from build123d import *

# Parameters (mm, degrees)
SKETCH_1_W             = 60
SKETCH_1_H             = 80
EXTRUDE_1_DEPTH        = 23
SKETCH_3_R             = 2
CUT_EXTRUDE_2_DEPTH    = 25
EXTRUDE_START          = -50
EXTRUDE_2_DEPTH        = 30
SKETCH_5_R             = 1.6
CUT_EXTRUDE_3_DEPTH    = 57.356011214
CUT_EXTRUDE_START      = -5
SKETCH_7_R             = 2
CUT_EXTRUDE_4_DEPTH    = 4.95
PATTERN_LINEAR_1_COUNT = 2
PATTERN_LINEAR_1_PITCH = 10


with BuildPart() as part:
    # 草图1 → 凸台-拉伸1 (new body)
    with BuildSketch(Plane.XY):
        Rectangle(SKETCH_1_W, SKETCH_1_H)
    extrude(amount=EXTRUDE_1_DEPTH)

    # 草图3 → 切除-拉伸2 (cut)
    with BuildSketch(Plane(origin=(0, 40, 0), x_dir=(1, 0, 0), z_dir=(0, 1, 0))):
        with Locations(Location((24.5, -6, 0), (0, 0, 270))):
            Circle(SKETCH_3_R)
        with Locations(Location((24.5, -16, 0), (0, 0, 270))):
            Circle(SKETCH_3_R)
    cut_extrude_2 = extrude(amount=-CUT_EXTRUDE_2_DEPTH, mode=Mode.SUBTRACT)

    # 镜向1: 切除-拉伸2 across plane
    add(cut_extrude_2.mirror(Plane(origin=(0, 0, 0), x_dir=(0, 0, 1), z_dir=(1, 0, 0))), mode=Mode.SUBTRACT)

    # 草图4 → 凸台-拉伸2 (add)
    with BuildSketch(Plane(origin=(0, 40, 0), x_dir=(1, 0, 0), z_dir=(0, 1, 0)).offset(EXTRUDE_START)):
        Polygon((13.575260778, -26), (10, -23), (0, -23), (0, -26), align=None)
        Polygon((0, -26), (0, -23), (-10, -23), (-13.575260778, -26), align=None)
    extrude(amount=-EXTRUDE_2_DEPTH)

    # 草图5 → 切除-拉伸3 (cut, through all)
    with BuildSketch(Plane(origin=(0, 0, 0), x_dir=(-1, 0, 0), z_dir=(0, 0, -1))):
        with Locations((-24.5, -25)):
            Circle(SKETCH_5_R)
        with Locations((24.5, -25)):
            Circle(SKETCH_5_R)
    extrude(amount=-CUT_EXTRUDE_3_DEPTH, mode=Mode.SUBTRACT)

    # 草图7 → 切除-拉伸4 (cut)
    # profile 1 of 3: a face of its own
    with BuildSketch(Plane(origin=(0, 40, 0), x_dir=(1, 0, 0), z_dir=(0, 1, 0)).offset(CUT_EXTRUDE_START)):
        Polygon((-26.491858429, -9.45), (-22.508141571, -9.45), (-20.516283143, -6), (-22.508141571, -2.55), (-26.491858429, -2.55), (-30, -2.55), (-30, -9.45), align=None)
        with Locations(Location((-24.5, -6, 0), (0, 0, 270))):
            Circle(SKETCH_7_R, mode=Mode.SUBTRACT)
    # profile 2 of 3: a face of its own
    with BuildSketch(Plane(origin=(0, 40, 0), x_dir=(1, 0, 0), z_dir=(0, 1, 0)).offset(CUT_EXTRUDE_START)):
        Polygon((26.491858429, -9.45), (28.483716857, -6), (26.491858429, -2.55), (22.508141571, -2.55), (20.516283143, -6), (22.508141571, -9.45), align=None)
        with Locations(Location((24.5, -6, 0), (0, 0, 270))):
            Circle(SKETCH_7_R, mode=Mode.SUBTRACT)
    # profile 3 of 3: a face of its own
    with BuildSketch(Plane(origin=(0, 40, 0), x_dir=(1, 0, 0), z_dir=(0, 1, 0)).offset(CUT_EXTRUDE_START)):
        Polygon((26.491858429, -9.45), (30, -9.45), (30, -2.55), (26.491858429, -2.55), (28.483716857, -6), align=None)
    cut_extrude_4 = extrude(amount=-CUT_EXTRUDE_4_DEPTH, mode=Mode.SUBTRACT)

    # 阵列(线性)1: 切除-拉伸4 ×2
    with Locations(*[(0, 0, i * PATTERN_LINEAR_1_PITCH) for i in range(1, PATTERN_LINEAR_1_COUNT)]):
        add(cut_extrude_4, mode=Mode.SUBTRACT)


solid = part.part
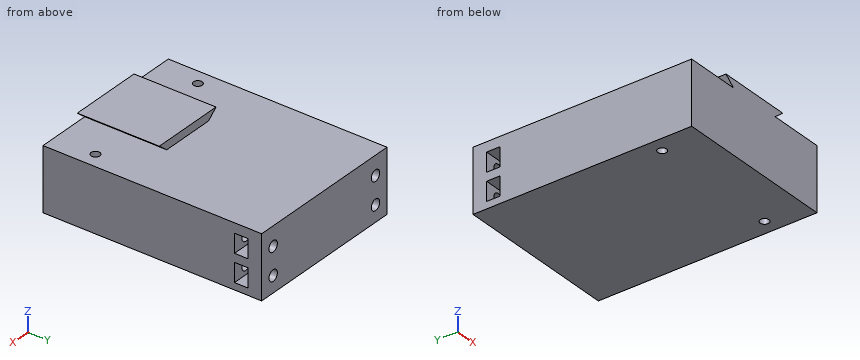
The listing builds one solid part. Answer for the finished solid, in the listing's coordinates (mm). Coordinates: 2 decimals unless noted, no trailing zeros. Write each loop counter-clockwise with the first axis right and the second up, starting at its lowest first coordinate (ties: lowest second). Pieces come first, ordered by that corner, then holes. Notation, with made-up numbers: (28.25, 45) -> (67.25, 45) arc R16 cw to (67.25, 51) -> close; hole circle Ø1 at (40.25, 66.5). An arc over 180 degrees is marked (long way). One line per question, with ' | ' between items.
1. Section A-A (z = 17) is taken. State how many separate pieces and enclosed holes the cut face has, and give its area (3 significant figures).
Verdict:
separate pieces: 3 | enclosed holes: 2 | area: 4,560 mm^2
2. Section C-C (y = -25) is taken. Determine the outline of the cut face in (x, z), and give its area (3 significant figures).
Verdict:
outline: (-30, 0) -> (-26.1, 0) -> (-26.1, 23) -> (-30, 23) -> close; (-22.9, 0) -> (22.9, 0) -> (22.9, 23) -> (10, 23) -> (13.58, 26) -> (-13.58, 26) -> (-10, 23) -> (-22.9, 23) -> close; (26.1, 0) -> (30, 0) -> (30, 23) -> (26.1, 23) -> close | area: 1,300 mm^2
3. Given pin 1 Ø1.2 at (x, z) = (24.5, 6.5) entering from +Y; pin 2 Ø8 at (x, y) = (22.5, 21) entering from +Z, each flat-ended and moving along its own axis, determine where each tip first touches the part or whether it passes through.
Verdict:
pin 1: stops at y = 15 | pin 2: stops at z = 23
4. Straight lines are drawn through the part: line 1 (X direction, y = 26.75, z = 6); line 2 (Z direction, x = -24.5, y = 27); line 3 (Z direction, x = 24, y = 36). For each, find the intervals that lie inside material, in ascending order.
Verdict:
line 1: x = -30 to -26.5, -22.5 to 22.5, 26.5 to 30 | line 2: z = 0 to 4, 8 to 14, 18 to 23 | line 3: z = 0 to 4.06, 7.94 to 14.06, 17.94 to 23
5. Section D-D (y = 27.5) is taken. Determine the outline of the cut face in (x, z), and give its area (3 significant figures).
Verdict:
outline: (-30, 0) -> (30, 0) -> (30, 23) -> (-30, 23) -> close; hole circle Ø4 at (-24.5, 6); hole circle Ø4 at (-24.5, 16); hole circle Ø4 at (24.5, 6); hole circle Ø4 at (24.5, 16) | area: 1,330 mm^2
